Here's how the part is built. I have some questions about the finished solid (model axes, mm). Face numbers are marked on the shaded views. A direction names the side the tool comes from. Give positions to 0.01 mm unless a question says otherwise; leave off trailing zeros. Write each loop counter-clockwise with the first axis right and the second up, starting at its lowest first coordinate (ties: lowest second). Pieces come first, ordered by that corner, then holes. Notation, with made-up numbers: (-28, -8) -> (17, -8) arc R12 cw to (17, 6) -> close; hole circle Ø1 at (80.5, -36). An arc over 180 degrees is marked (long way). Return JSON: item names as keys, results as strings.
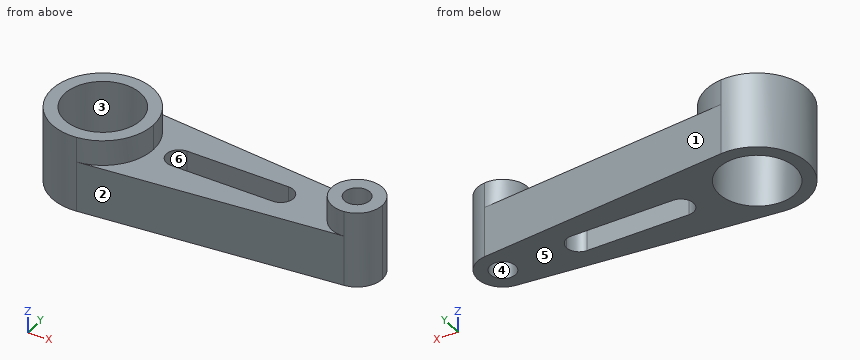
from build123d import *

# Parameters (mm, degrees)
F1_DEPTH = 25.4
F0_R     = 19.05
F0_R_2   = 6.35
F2_DEPTH = 38.1


with BuildPart() as f1:
    # F0 (on Top) → F1 (new body)
    with BuildSketch(Plane.XY):
        with BuildLine():
            ThreePointArc((110.078714, -12.636359), (96.108901, 4.5e-05), (110.078804, 12.63635))
            Line((110.078804, 12.63635), (-15.665499, 25.273153))
            ThreePointArc((-15.665499, 25.273153), (0.631774, 17.039363), (7.194695, 0.000453))
            ThreePointArc((7.194695, 0.000453), (0.631713, -17.038525), (-15.665679, -25.272266))
            Line((-15.665679, -25.272266), (110.078714, -12.636359))
        make_face()
        with BuildLine():
            ThreePointArc((70.708901, 6.35), (75.199029, 4.490128), (77.058901, 0))
            ThreePointArc((77.058901, 0), (75.199029, -4.490128), (70.708901, -6.35))
            Line((70.708901, -6.35), (19.908901, -6.35))
            ThreePointArc((19.908901, -6.35), (13.558901, 0), (19.908901, 6.35))
            Line((19.908901, 6.35), (70.708901, 6.35))
        make_face(mode=Mode.SUBTRACT)
    extrude(amount=F1_DEPTH)

    # F0 (on Top) → F2 (join)
    with BuildSketch(Plane.XY):
        with BuildLine():
            ThreePointArc((7.194695, 0.000453), (0.631774, 17.039363), (-15.665499, 25.273153))
            ThreePointArc((-15.665499, 25.273153), (-43.605305, 0.000543), (-15.665679, -25.272266))
            ThreePointArc((-15.665679, -25.272266), (0.631713, -17.038525), (7.194695, 0.000453))
        make_face()
        with Locations((-18.205305, 0.000453)):
            Circle(F0_R, mode=Mode.SUBTRACT)
        with BuildLine():
            ThreePointArc((110.078714, -12.636359), (118.22741, -8.519489), (121.508901, 0))
            ThreePointArc((121.508901, 0), (118.22744, 8.519455), (110.078804, 12.63635))
            ThreePointArc((110.078804, 12.63635), (96.108901, 4.5e-05), (110.078714, -12.636359))
        make_face()
        with Locations((108.808901, 0)):
            Circle(F0_R_2, mode=Mode.SUBTRACT)
    extrude(amount=F2_DEPTH)


solid = f1.part
1. Suppose I cut it at D-D, the plane y = 2.5. List the corners of the cut face in (x, z) for me, and give its area (3 significant figures).
Taken from the geometry:
{"outline": "(-43.48, 0) -> (-37.09, 0) -> (-37.09, 38.1) -> (-43.48, 38.1) -> close; (0.68, 0) -> (14.07, 0) -> (14.07, 25.4) -> (7.07, 25.4) -> (7.07, 38.1) -> (0.68, 38.1) -> close; (76.55, 0) -> (102.97, 0) -> (102.97, 38.1) -> (96.36, 38.1) -> (96.36, 25.4) -> (76.55, 25.4) -> close; (114.65, 0) -> (121.26, 0) -> (121.26, 38.1) -> (114.65, 38.1) -> close", "area": "1,670 mm²"}
2. If we mould it in two halves opening along Y, with no side actions, what happens to the marked faces 1, 2, 3 and 4? For each: released by +Y, released by -Y, zero draft, split by the parting line, or undercut.
Taken from the geometry:
{"face 1": "released by +Y", "face 2": "released by -Y", "face 3": "undercut", "face 4": "undercut"}
3. If I drill on line 1 (X direction, y = 2, z = 4); line 2 (X direction, y = -3, z = 30); line 3 (Y direction, x = -30, z = 3) (3 decimals), over which ranges is the centre line in solid material (lowest first)? Write a range as [from, to].
Taken from the geometry:
{"line 1": "x = [-43.53, -37.15], [0.74, 13.88], [76.74, 102.78], [114.84, 121.35]", "line 2": "x = [-43.43, -37.02], [0.61, 7.02], [96.47, 103.21], [114.41, 121.15]", "line 3": "y = [-22.495, -14.959], [14.96, 22.496]"}
4. Suppose I cut it at A-A, the plane z = 31. List the corners of the cut face in (x, y) for me, and give its area (3 significant figures).
Taken from the geometry:
{"outline": "circle Ø50.8 at (-18.21, 0); (110.08, -12.64) arc R12.7 ccw to (121.51, 0) arc R12.7 ccw (long way) to start; hole circle Ø38.1 at (-18.21, 0); hole circle Ø12.7 at (108.81, 0)", "area": "1,270 mm²"}
5. Which directions (+Z, -Z, +X, -X, +Y, -Y) give clear straight access to the entire face, cutting with the end or side of a thin tool? Please do the marked faces 5 and 6.
Taken from the geometry:
{"face 5": "-Z, +X, -X, +Y, -Y", "face 6": "+Z, -Z"}
6. For pin 1 Ø4 at (x, y) = (26.5, 14.5) entering from +Z; pin 2 Ø6 at (x, z) = (56.5, 28.5) entering from +Y; pin 3 Ø5 at (x, z) = (-22, 9) entering from -Y; pin 4 Ø7.5 at (x, z) = (37, 10.5) entering from +Y, each with a flat end and sliding along its axis, tell me the tip position at first contact or that it passes through.
Taken from the geometry:
{"pin 1": "stops at z = 25.4", "pin 2": "passes through", "pin 3": "stops at y = -25.37", "pin 4": "stops at y = 20.36"}
7. Suppose I cut it at C-C, the plane y = 15. List the corners of the cut face in (x, z) for me, and give its area (3 significant figures).
Taken from the geometry:
{"outline": "(-38.7, 0) -> (-29.95, 0) -> (-29.95, 38.1) -> (-38.7, 38.1) -> close; (-6.46, 0) -> (86.56, 0) -> (86.56, 25.4) -> (2.29, 25.4) -> (2.29, 38.1) -> (-6.46, 38.1) -> close", "area": "2,810 mm²"}
8. Suppose I cut it at B-B, the plane x = 45. List the corners of the cut face in (y, z) for me.
Taken from the geometry:
{"outline": "(-19.18, 0) -> (-6.35, 0) -> (-6.35, 25.4) -> (-19.18, 25.4) -> close; (6.35, 0) -> (19.18, 0) -> (19.18, 25.4) -> (6.35, 25.4) -> close"}
